Check sheet for the drawn part. Datum: minimum x, y, z corner. Units: mm. Coordinates: 2 decimals unless noted, no trailing zeros. Write each loop counter-clockwise with the first axis right and the second up, starting at its lowest first coordinate (ties: lowest second). Pieces come first, ordered by that corner, then holes. Notation, with made-up numbers: M 43,-29 L 96,-29 A15 ccw 96,-14 Z; hole C 4.5,5 d9. An arc over 180 degrees is marked long. Answer as CSV lines item,"result".
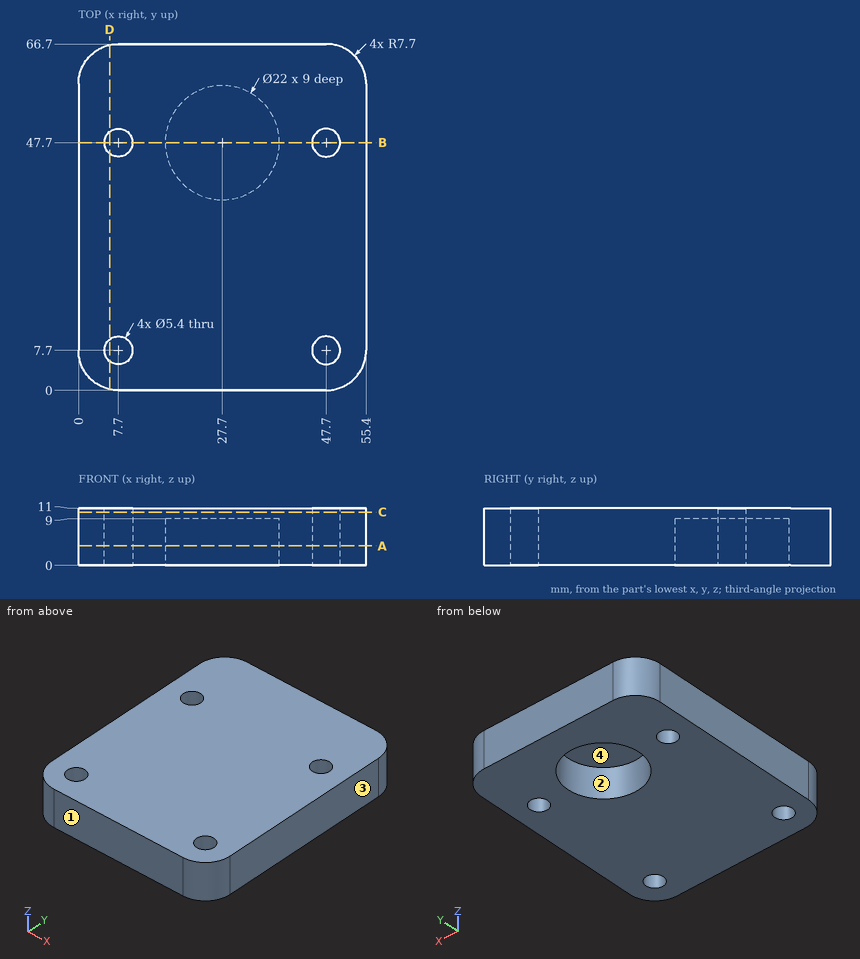
1) Section check B-B, the plane y = 47.7. Record the boundary of the cut face in (x, z), plus the area to 3 significant figures.
Answer key:
outline,"M 0,0 L 5,0 L 5,11 L 0,11 Z; M 10.4,0 L 16.7,0 L 16.7,9 L 38.7,9 L 38.7,0 L 45,0 L 45,11 L 10.4,11 Z; M 50.4,0 L 55.4,0 L 55.4,11 L 50.4,11 Z"
area,"293 mm2"
2) Section check C-C, the plane z = 10.25. Record the boundary of the cut face in (x, y).
Answer key:
outline,"M 0,7.7 A7.7 ccw 7.7,0 L 47.7,0 A7.7 ccw 55.4,7.7 L 55.4,59 A7.7 ccw 47.7,66.7 L 7.7,66.7 A7.7 ccw 0,59 Z; hole C 7.7,7.7 d5.4; hole C 7.7,47.7 d5.4; hole C 47.7,7.7 d5.4; hole C 47.7,47.7 d5.4"
3) Section check D-D, the plane x = 6. Record the boundary of the cut face in (y, z), plus the area to 3 significant figures.
Answer key:
outline,"M 0.19,0 L 5.6,0 L 5.6,11 L 0.19,11 Z; M 9.8,0 L 45.6,0 L 45.6,11 L 9.8,11 Z; M 49.8,0 L 66.51,0 L 66.51,11 L 49.8,11 Z"
area,"637 mm2"
4) Depth check by flat-ended pin: P1, Ø5, axis at y = 59.5, z = 6, coming from the -X side; P2, Ø6.5, axis at x = 28, y = 44.5, coming from the -Z side. Enter the tip coordinate at first touch or a pass-through.
Answer key:
P1,"stops at x = 0"
P2,"stops at z = 9"
5) Section check A-A, the plane z = 3.75. Record the boundary of the cut face in (x, y).
Answer key:
outline,"M 0,7.7 A7.7 ccw 7.7,0 L 47.7,0 A7.7 ccw 55.4,7.7 L 55.4,59 A7.7 ccw 47.7,66.7 L 7.7,66.7 A7.7 ccw 0,59 Z; hole C 7.7,7.7 d5.4; hole C 7.7,47.7 d5.4; hole C 27.7,47.7 d22; hole C 47.7,7.7 d5.4; hole C 47.7,47.7 d5.4"
6) Thickness scan on line 1 along Y through (x, z) = (47.7, 4.5); line 2 along Y through (x, z) = (27.7, 4); line 3 along X through (y, z) = (49, 4). Record the ranges inside material, lowest first.
Answer key:
line 1,"y = 0 to 5, 10.4 to 45, 50.4 to 66.7"
line 2,"y = 0 to 36.7, 58.7 to 66.7"
line 3,"x = 0 to 5.33, 10.07 to 16.78, 38.62 to 45.33, 50.07 to 55.4"
7) Mould release check, pull along X, two halves, no side actions. Record for the marked faces 1, 2, 3 and 4: pulls with the +X half, pulls with the -X half, needs draft (parallel to the pull), parting line crosses it, or undercut.
Answer key:
face 1,"needs draft"
face 2,"undercut"
face 3,"pulls with the +X half"
face 4,"undercut"
